The model under review builds one solid part; all positions refer to its coordinate system, in mm. A direction names the side the tool comes from. Coordinates: 2 decimals unless noted, no trailing zeros. Loops run counter-clockwise (first coordinate to the right, second up) from the corner with the lowest first, then second, coordinate; pieces in that order, holes last. Notation, with made-up numbers: M -9.75,64 L 28.25,64 A20 ccw 28.25,100 Z; hole C 58.5,53 d4. An arc over 180 degrees is marked long. One line per item, written item: value.
```python
from build123d import *

# Parameters (mm, degrees)
ESQUISSE1_W                  = 350
ESQUISSE1_H                  = 350
BOSS_EXTRU_1_DEPTH           = 26
ESQUISSE2_W                  = 350
ESQUISSE2_H                  = 350
ESQUISSE2_W_2                = 298
ESQUISSE2_H_2                = 298
ENL_V_MAT_EXTRU_1_DEPTH      = 20
ESQUISSE3_W                  = 294
ESQUISSE3_H                  = 294
ENL_V_MAT_EXTRU_2_DEPTH      = 20
ENL_V_MAT_EXTRU_3_DEPTH      = 249.849352018
ENL_V_MAT_EXTRU_3_DEPTH_BACK = 249.849352018
ESQUISSE5_R                  = 6.5


with BuildPart() as part:
    # Esquisse1 → Boss.-Extru.1 (new body)
    with BuildSketch(Plane.XY):
        Rectangle(ESQUISSE1_W, ESQUISSE1_H)
    extrude(amount=BOSS_EXTRU_1_DEPTH)

    # Esquisse2 → Enlèv. mat.-Extru.1 (cut)
    with BuildSketch(Plane.XY.offset(26)):
        Rectangle(ESQUISSE2_W, ESQUISSE2_H)
        Rectangle(ESQUISSE2_W_2, ESQUISSE2_H_2, mode=Mode.SUBTRACT)
    extrude(amount=-ENL_V_MAT_EXTRU_1_DEPTH, mode=Mode.SUBTRACT)

    # Esquisse3 → Enlèv. mat.-Extru.2 (cut)
    with BuildSketch(Plane.XY.offset(26)):
        Rectangle(ESQUISSE3_W, ESQUISSE3_H)
    extrude(amount=-ENL_V_MAT_EXTRU_2_DEPTH, mode=Mode.SUBTRACT)

    # Esquisse5 → Enlèv. mat.-Extru.3 (cut, two sides: drawn at the far end of the back side and taken through both)
    with BuildSketch(Plane(origin=(0, 0, 0), x_dir=(-1, 0, 0), z_dir=(0, 0, -1)).offset(-ENL_V_MAT_EXTRU_3_DEPTH_BACK)):
        with Locations((-50, 111.5)):
            Circle(ESQUISSE5_R)
        with Locations((50, 111.5)):
            Circle(ESQUISSE5_R)
        with Locations((50, -111.5)):
            Circle(ESQUISSE5_R)
        with Locations((-50, -111.5)):
            Circle(ESQUISSE5_R)
    extrude(amount=ENL_V_MAT_EXTRU_3_DEPTH + ENL_V_MAT_EXTRU_3_DEPTH_BACK, mode=Mode.SUBTRACT)


solid = part.part
```
(1) Add section A-A on x = 50. State the section outline as (y, z) points.
Checks:
outline: M -175,0 L -118,0 L -118,6 L -147,6 L -147,26 L -149,26 L -149,6 L -175,6 Z; M -105,0 L 105,0 L 105,6 L -105,6 Z; M 118,0 L 175,0 L 175,6 L 149,6 L 149,26 L 147,26 L 147,6 L 118,6 Z
(2) Add section D-D on y = -36. State the section outline as (x, z) points, then the cut area to 3 significant figures.
Checks:
outline: M -175,0 L 175,0 L 175,6 L 149,6 L 149,26 L 147,26 L 147,6 L -147,6 L -147,26 L -149,26 L -149,6 L -175,6 Z
area: 2,180 mm^2
(3) Tool access review of faces 1 (the face through (-2, -149, 16)), 2 (the face through (-2, -147, 16)), 3 (the face through (-2, 149, 16)): name each direction out of +Z, -Z, +X, -X, +Y, -Y from which nothing blocks a thin tool from reaching the whole face with its end or side.
Checks:
face 1: +Z, +X, -X, -Y
face 2: +Z
face 3: +Z, +X, -X, +Y
(4) Insertion check: pin 1 Ø17 at (x, y) = (50, 111.5) entering from +Z; pin 2 Ø10 at (y, z) = (4, 16.5) entering from +X; pin 3 Ø1 at (y, z) = (-136.5, 10.5) entering from -X. Each pin has a flat end and moves straight along its axis. Give the tip position at first contact, or say it passes through.
Checks:
pin 1: z = 6
pin 2: x = 149
pin 3: x = -149
(5) Add section C-C on y = 111.5. State the section outline as (x, z) points, then the cut area to 3 significant figures.
Checks:
outline: M -175,0 L -56.5,0 L -56.5,6 L -147,6 L -147,26 L -149,26 L -149,6 L -175,6 Z; M -43.5,0 L 43.5,0 L 43.5,6 L -43.5,6 Z; M 56.5,0 L 175,0 L 175,6 L 149,6 L 149,26 L 147,26 L 147,6 L 56.5,6 Z
area: 2,020 mm^2
(6) Add section B-B on z = 16. State the section outline as (x, y) points.
Checks:
outline: M -149,-149 L 149,-149 L 149,149 L -149,149 Z; hole M -147,-147 L 147,-147 L 147,147 L -147,147 Z
(7) Draft analysis for pull direction X (two halves, no side actions). For faces 4 (the face through (56.494, 111.786, 3.042)), 5 (the face through (-2, 147, 16)), 6 (the face through (-149, -2, 16)), 7 (the face through (153, 2, 6)), state which applies: pulls with the +X half, pulls with the -X half, needs draft (parallel to the pull), parting line crosses it, or undercut.
Checks:
face 4: undercut
face 5: undercut
face 6: pulls with the -X half
face 7: needs draft
(8) To check wall thickness, follow L1, parallel to X at y = -111.5, z = 2.85; L2, parallel to Y at x = 50, z = 4.5; L3, parallel to X at y = -78, z = 12. State the ranges of each line that lie inside material, in increasing order. Write a range as [from, to].
Checks:
L1: [-175, -56.5], [-43.5, 43.5], [56.5, 175]
L2: [-175, -118], [-105, 105], [118, 175]
L3: [-149, -147], [147, 149]
